from build123d import *

# Parameters (mm, degrees)
BOSS_EXTRUDE1_DEPTH = 40
SKETCH5_R           = 3.5
BOSS_EXTRUDE2_DEPTH = 8.091605471
SKETCH5_2_R         = 3.5
BOSS_EXTRUDE3_DEPTH = 8
BOSS_EXTRUDE6_START = 8
SKETCH9_R           = 3.5
BOSS_EXTRUDE6_DEPTH = 8


with BuildPart() as part:
    # Sketch3 → Boss-Extrude1 (new body)
    with BuildSketch(Plane(origin=(0, 0, 0), x_dir=(1, 0, 0), z_dir=(0, 1, 0))):
        Polygon((-5.773502692, 0), (-2.886751346, -5), (2.886751346, -5), (5.773502692, 0), (2.886751346, 5), (-2.886751346, 5), align=None)
    extrude(amount=BOSS_EXTRUDE1_DEPTH)

    # Sketch5 → Boss-Extrude2 (add)
    with BuildSketch(Plane(origin=(0, 40, 0), x_dir=(1, 0, 0), z_dir=(0, 1, 0))):
        with Locations(Location((0, 0, 0), (0, 0, 270))):
            Circle(SKETCH5_R)
    extrude(amount=BOSS_EXTRUDE2_DEPTH)

    # Sketch5_2 → Boss-Extrude3 (add)
    with BuildSketch(Plane(origin=(0, 40, 0), x_dir=(1, 0, 0), z_dir=(0, 1, 0))):
        with Locations(Location((0, 0, 0), (0, 0, 270))):
            Circle(SKETCH5_2_R)
    extrude(amount=BOSS_EXTRUDE3_DEPTH)

    # Sketch9 → Boss-Extrude6 (add)
    with BuildSketch(Plane.XZ.offset(BOSS_EXTRUDE6_START)):
        with Locations(Location((0, 0, 0), (0, 0, 90))):
            Circle(SKETCH9_R)
    extrude(amount=-BOSS_EXTRUDE6_DEPTH)


solid = part.part
For this review, take the finished solid that the model builds, in its own axes (mm). A direction names the side the tool comes from. Coordinates: 2 decimals unless noted, no trailing zeros. Loops run counter-clockwise (first coordinate to the right, second up) from the corner with the lowest first, then second, coordinate; pieces in that order, holes last. Notation, with made-up numbers: (50, -12) - (90, -12) arc R13 cw to (90, -5) - close; hole circle Ø4 at (75, 86.5). An arc over 180 degrees is marked (long way). Return JSON: item names as keys, results as strings.
Item 1: Take a section at B-B (z = -1.5). Give the boundary of the cut face in (x, y), then the cut area to 3 significant figures.
Determined:
{"outline": "(-4.91, 0) - (-3.16, 0) - (-3.16, -8) - (3.16, -8) - (3.16, 0) - (4.91, 0) - (4.91, 40) - (3.16, 40) - (3.16, 48.09) - (-3.16, 48.09) - (-3.16, 40) - (-4.91, 40) - close", "area": "494 mm2"}
Item 2: For line 1 (Y direction, x = 2, z = -3.25); line 2 (Z direction, x = 0.25, y = 43); line 3 (X direction, y = 21.5, z = 2), list the stretches that pass through material, from the lowest coordinate up.
Determined:
{"line 1": "y = 0 to 40", "line 2": "z = -3.49 to 3.49", "line 3": "x = -4.62 to 4.62"}
Item 3: Take a section at D-D (x = 4.5). Give the boundary of the cut face in (y, z).
Determined:
{"outline": "(0, -2.21) - (40, -2.21) - (40, 2.21) - (0, 2.21) - close"}
Item 4: Take a section at C-C (y = 25). Give the boundary of the cut face in (x, z).
Determined:
{"outline": "(-5.77, 0) - (-2.89, -5) - (2.89, -5) - (5.77, 0) - (2.89, 5) - (-2.89, 5) - close"}
Item 5: Take a section at A-A (x = 0). Give the boundary of the cut face in (y, z), then the cut area to 3 significant figures.
Determined:
{"outline": "(-8, -3.5) - (0, -3.5) - (0, -5) - (40, -5) - (40, -3.5) - (48.09, -3.5) - (48.09, 3.5) - (40, 3.5) - (40, 5) - (0, 5) - (0, 3.5) - (-8, 3.5) - close", "area": "513 mm2"}
Item 6: For faces 1 (the flat face through (4.35, 19.72, -2.465)), 2 (the flat face through (4, 0, 0)), 3 (the cylindrical face through (-3.417, 43.989, -0.759)), list the 3-axis set-ups (+Z, -Z, +X, -X, +Y, -Y) from which the entire face can be reached by the end or side of a thin tool; tool diameter is ignored.
Determined:
{"face 1": "-Z, +X, +Y, -Y", "face 2": "-Y", "face 3": "+Y"}
Item 7: Insertion check: pin 1 (3 mm diameter, centred on y = 19, z = 2.5, fed in from -X); pin 2 (5 mm diameter, centred on x = 3.5, z = -0.5, fed in from +Y); pin 3 (1 mm diameter, centred on x = -3.5, y = 28, fed in from +Z); pin 4 (6 mm diameter, centred on y = 16, z = 0.5, fed in from +X). Each pin has a flat end and moves straight along its axis. Give the tip position at first contact, or say it passes through.
Determined:
{"pin 1": "stops at x = -5.2", "pin 2": "stops at y = 48.09", "pin 3": "stops at z = 4.8", "pin 4": "stops at x = 5.77"}
